For this review, take the finished solid that the model builds, in its own axes (mm). A direction names the side the tool comes from. Give positions to 0.01 mm unless a question says otherwise; leave off trailing zeros. Order: outer loops, then holes, each group sorted by start corner. A loop starts at its lowest first (then second) coordinate and runs counter-clockwise, first axis right, second up. Notation, with made-up numbers: (19, 30) -> (28, 30) arc R27 cw to (28, 68) -> close; hole circle Ø1 at (-22, 61.5). An arc over 180 degrees is marked (long way). Return JSON: item names as keys, results as strings. Group by question number.
1) Insertion check: P1, Ø1.8, axis at y = 15.5, z = 0.5, coming from the +X side; P2, Ø1.8, axis at y = 15, z = 1.5, coming from the -X side; P3, Ø6, axis at x = -3, y = 9.5, coming from the +Z side; P4, Ø1.5, axis at x = 1.5, y = 1.5, coming from the -Z side. Each pin has a flat end and moves straight along its axis. Give the tip position at first contact, or say it passes through.
2) For faces 1 (the face through (3, 6, 0)), 2 (the face through (-0.95, 15, 0)), 3 (the face through (-3, 16, 0)), list the 3-axis set-ups (+Z, -Z, +X, -X, +Y, -Y) from which the entire face can be reached by the end or side of a thin tool; tool diameter is ignored.
3) The part is to be moulded in two halves that separate along X. For faces 4 (the face through (-1.44, 12.82, 2.77)), 5 (the face through (0, 14.4, 0)), 6 (the face through (3, 16, 0)), 7 (the face through (0.95, 15, 0)), say which applies: released by +X, released by -X, zero draft, split by the parting line, or undercut.
4) To check wall thickness, follow line 1 along Y through (x, z) = (-1.25, -0.5); line 2 along Z through (x, y) = (2.75, 7.75); line 3 along Z through (x, y) = (1.75, 15). State the ranges of each line that lie inside material, in increasing order.
5) Add section A-A (y = 9.5). Give the boundary of the cut face in (x, z), then the cut area to 3 significant figures.
from build123d import *

# Parameters (mm, degrees)
CUT_EXTRUDE1_DEPTH      = 18.759645267
CUT_EXTRUDE1_DEPTH_BACK = 18.759645267
SKETCH2_W               = 1.9
SKETCH2_H               = 1.6


with BuildPart() as part:
    # Sketch1 → Revolve1 (revolve)
    with BuildSketch(Plane.XY):
        Polygon((0, 16), (-5.45, 16), (-5.45, 15.15), (-3, 12.7), (-3, 0), (0, -1.732050808), align=None)
    revolve(axis=Axis((0, 16, 0), (0, -1, 0)))

    # Sketch2 → Cut-Extrude1 (cut, two sides: drawn at the far end of the back side and taken through both)
    with BuildSketch(Plane.XY.offset(-CUT_EXTRUDE1_DEPTH_BACK)):
        with Locations((0, 15.2)):
            Rectangle(SKETCH2_W, SKETCH2_H)
    extrude(amount=CUT_EXTRUDE1_DEPTH + CUT_EXTRUDE1_DEPTH_BACK, mode=Mode.SUBTRACT)


solid = part.part
Evaluation:
{
 "1": {"P1": "x = 5.45", "P2": "x = -5.42", "P3": "z = 3", "P4": "z = -2.9"},
 "2": {"face 1": "-Y", "face 2": "+Z, -Z, +Y", "face 3": "+Z, -Z, +X, -X, +Y"},
 "3": {"face 4": "split by the parting line", "face 5": "undercut", "face 6": "zero draft", "face 7": "undercut"},
 "4": {"line 1": "-0.95 to 16", "line 2": "-1.2 to 1.2", "line 3": "-5 to 5"},
 "5": {"outline": "circle Ø6 at (0, 0)", "area": "28.3 mm^2"}
}
